from build123d import *

# Parameters (mm, degrees)
SKETCH_1_R      = 27.5
EXTRUDE_1_DEPTH = 2
SKETCH_2_R      = 27.5
SKETCH_2_R_2    = 25
EXTRUDE_2_DEPTH = 12
SKETCH_3_R      = 5
EXTRUDE_3_DEPTH = 40
CHAMFER_2_SIZE  = 3
CHAMFER_3_SIZE  = 3
FILLET_3_R      = 5


with BuildPart() as part:
    # 草图1 → 凸台-拉伸1 (new body)
    with BuildSketch(Plane.XY):
        Circle(SKETCH_1_R)
    extrude(amount=EXTRUDE_1_DEPTH)

    # 草图2 → 凸台-拉伸2 (add)
    with BuildSketch(Plane.XY.offset(2)):
        Circle(SKETCH_2_R)
        Circle(SKETCH_2_R_2, mode=Mode.SUBTRACT)
    extrude(amount=EXTRUDE_2_DEPTH)

    # 草图3 → 凸台-拉伸3 (add)
    with BuildSketch(Plane.XY.offset(2)):
        Circle(SKETCH_3_R)
    extrude(amount=EXTRUDE_3_DEPTH)

    # 倒角2
    chamfer_2_edges = [part.edges().sort_by_distance(p)[0] for p in [
        (-25, 0, 2),
    ]]
    chamfer(chamfer_2_edges, length=CHAMFER_2_SIZE)

    # 倒角3
    chamfer_3_edges = [part.edges().sort_by_distance(p)[0] for p in [
        (-5, 0, 2),
    ]]
    chamfer(chamfer_3_edges, length=CHAMFER_3_SIZE)

    # 圆角3
    fillet_3_edges = [part.edges().sort_by_distance(p)[0] for p in [
        (-5, 0, 42),
    ]]
    fillet(fillet_3_edges, radius=FILLET_3_R)


solid = part.part
For this review, take the finished solid that the model builds, in its own axes (mm). Give positions to 0.01 mm unless a question says otherwise; leave off trailing zeros. Order: outer loops, then holes, each group sorted by start corner. A loop starts at its lowest first (then second) coordinate and runs counter-clockwise, first axis right, second up. Notation, with made-up numbers: (14, 38.5) - (57, 38.5) arc R20 ccw to (57, 47.5) - close; hole circle Ø9 at (32, 17). An arc over 180 degrees is marked (long way). Answer as a JSON object with one key per item and string values. Group by question number.
Item 1: Clearance check with flat-ended pins moving along their axes: pin 1 Ø2 at (x, z) = (-9, 4.5) entering from -Y; pin 2 Ø1 at (x, y) = (-8, 9.5) entering from +Z; pin 3 Ø10 at (y, z) = (2, 30.5) entering from -X. State where each tip first meets the part, or that it passes through.
Item 2: Wall thickness on line 1 along Y through (x, z) = (0, 12); line 2 along X through (y, z) = (1.5, 3.5); line 3 along Z through (x, y) = (-15.5, -3): over which ranges is each line inside the solid? List them lowest first.
Item 3: Take a section at A-A on y = 0. Give the boundary of the cut face in (x, z), and give its area (3 significant figures).
Item 4: Take a section at B-B on z = 10.5. Give the boundary of the cut face in (x, y), and give its area (3 significant figures).
Item 5: Take a section at D-D on z = 19.5. Give the boundary of the cut face in (x, y), and give its area (3 significant figures).
Item 6: Draft analysis for pull direction Y (two halves, no side actions). For faces 1 (the cylindrical face through (-5.961, -26.846, 6.902)), 2 (the conical face through (-4.801, -21.619, 2.146)), 3 (the flat face through (0, 0, 0)), state which applies: pulls with the +Y half, pulls with the -Y half, needs draft (parallel to the pull), parting line crosses it, or undercut.
Reported:
{
 "1": {"pin 1": "y = -26.31", "pin 2": "z = 2", "pin 3": "x = -5"},
 "2": {"line 1": "-27.5 to -25, -5 to 5, 25 to 27.5", "line 2": "-27.46 to -23.45, -6.32 to 6.32, 23.45 to 27.46", "line 3": "0 to 2"},
 "3": {"outline": "(-27.5, 0) - (27.5, 0) - (27.5, 14) - (25, 14) - (25, 5) - (22, 2) - (8, 2) - (5, 5) - (5, 37) arc R5 ccw to (-5, 37) - (-5, 5) - (-8, 2) - (-22, 2) - (-25, 5) - (-25, 14) - (-27.5, 14) - close", "area": "577 mm^2"},
 "4": {"outline": "circle Ø55 at (0, 0); circle Ø10 at (0, 0); hole circle Ø50 at (0, 0)", "area": "491 mm^2"},
 "5": {"outline": "circle Ø10 at (0, 0)", "area": "78.5 mm^2"},
 "6": {"face 1": "parting line crosses it", "face 2": "undercut", "face 3": "needs draft"}
}
